from build123d import *

# Parameters (mm, degrees)
F1_DEPTH = 10.16
F3_DEPTH = 7.62


# Not quite as in the source:
# - a feature names something its author has since deleted; it is built from what else it names


with BuildPart() as f1:
    # F0 (on Top) → F1 (new body)
    with BuildSketch(Plane.XY):
        Polygon((-19.05, 19.05), (0, 0), (0, 5.2605122421), (0, 38.1), align=None)
        with BuildLine():
            Line((1.1407175417, 0), (0, 0))
            Line((0, 0), (0, -38.1))
            Line((0, -38.1), (19.05, -19.05))
            Line((19.05, -19.05), (3.7197438789, -3.7197438789))
            ThreePointArc((3.7197438789, -3.7197438789), (2.263176494, -1.9756963719), (1.1407175417, 0))
        make_face()
        Polygon((-19.05, -19.05), (0, 0), (-38.1, 0), align=None)
        Polygon((-38.1, 0), (0, 0), (-19.05, 19.05), align=None)
        Polygon((0, -38.1), (0, 0), (-19.05, -19.05), align=None)
        with BuildLine():
            Line((0, 38.1), (0, 5.2605122421))
            ThreePointArc((0, 5.2605122421), (0.2032791438, 2.9973357481), (0.8066091092, 0.8066091092))
            Line((0.8066091092, 0.8066091092), (19.05, 19.05))
            Line((19.05, 19.05), (0, 38.1))
        make_face()
        with BuildLine():
            ThreePointArc((0.8066091092, 0.8066091092), (0.9667299371, 0.4004326511), (1.1407175417, 0))
            Line((1.1407175417, 0), (38.1, 0))
            Line((38.1, 0), (19.05, 19.05))
            Line((19.05, 19.05), (0.8066091092, 0.8066091092))
        make_face()
        with BuildLine():
            Line((38.1, 0), (1.1407175417, 0))
            ThreePointArc((1.1407175417, 0), (2.263176494, -1.9756963719), (3.7197438789, -3.7197438789))
            Line((3.7197438789, -3.7197438789), (19.05, -19.05))
            Line((19.05, -19.05), (38.1, 0))
        make_face()
        Polygon((7.62, -45.72), (0, -38.1), (0, -63.5), align=None)
        Polygon((-7.62, -45.72), (0, -38.1), (-19.05, -19.05), align=None)
        Polygon((19.05, -19.05), (0, -38.1), (7.62, -45.72), align=None)
        Polygon((0, -63.5), (0, -38.1), (-7.62, -45.72), align=None)
        Polygon((-45.72, -7.62), (-38.1, 0), (-63.5, 0), align=None)
        Polygon((-45.72, 7.62), (-38.1, 0), (-19.05, 19.05), align=None)
        Polygon((-63.5, 0), (-38.1, 0), (-45.72, 7.62), align=None)
        Polygon((-19.05, -19.05), (-38.1, 0), (-45.72, -7.62), align=None)
        Polygon((-7.62, 45.72), (-19.05, 19.05), (0, 38.1), align=None)
        Polygon((-7.62, 45.72), (0, 38.1), (0, 63.5), align=None)
        Polygon((7.62, 45.72), (0, 38.1), (19.05, 19.05), align=None)
        Polygon((0, 63.5), (0, 38.1), (7.62, 45.72), align=None)
        Polygon((45.72, 7.62), (38.1, 0), (63.5, 0), align=None)
        Polygon((45.72, -7.62), (38.1, 0), (19.05, -19.05), align=None)
        Polygon((19.05, 19.05), (38.1, 0), (45.72, 7.62), align=None)
        Polygon((63.5, 0), (38.1, 0), (45.72, -7.62), align=None)
        Polygon((7.62, -45.72), (0, -63.5), (-7.62, -45.72), (-25.4, -63.5), (0, -75.1397422652), (25.4, -63.5), align=None)
        Polygon((-45.72, -7.62), (-63.5, 0), (-45.72, 7.62), (-63.5, 25.4), (-75.1397422652, 0), (-63.5, -25.4), align=None)
        Polygon((-25.4, 63.5), (-7.62, 45.72), (0, 63.5), (7.62, 45.72), (25.4, 63.5), (0, 75.1238912344), align=None)
        Polygon((45.72, 7.62), (63.5, 0), (45.72, -7.62), (63.5, -25.4), (75.1397422652, 0), (63.5, 25.4), align=None)
    extrude(amount=F1_DEPTH)

    # F2 (on face) → F3 (join)
    with BuildSketch(Plane.XY.offset(10.16)):
        Polygon((-19.05, 19.05), (-45.72, 7.62), (-45.72, -7.62), (-19.05, -19.05), (-7.62, -45.72), (7.62, -45.72), (19.05, -19.05), (45.72, -7.62), (45.72, 7.62), (19.05, 19.05), (7.62, 45.72), (-7.62, 45.72), align=None)
        Polygon((0, -30.48), (-30.48, 0), (0, 30.48), (30.48, 0), align=None, mode=Mode.SUBTRACT)
    extrude(amount=F3_DEPTH)


solid = f1.part
Input: part model. Units: mm. Frame: model coordinates. A direction names the side the tool comes from. Give positions to 0.01 mm unless a question says otherwise; leave off trailing zeros. Order: outer loops, then holes, each group sorted by start corner. A loop starts at its lowest first (then second) coordinate and runs counter-clockwise, first axis right, second up. Notation, with made-up numbers: (87, 69.25) - (116, 69.25) arc R23 cw to (116, 92.25) - close; hole circle Ø1 at (86.5, -1). An arc over 180 degrees is marked (long way). Write each question's results on one line, items separated by ' | '.
Item 1: Contact query for flat-ended pins moving along their axis: pin 1 Ø6 at (y, z) = (1.5, 3.5) entering from +X; pin 2 Ø10 at (x, y) = (-16, -2) entering from +Z; pin 3 Ø2.5 at (y, z) = (0.5, 15) entering from +X; pin 4 Ø2 at (x, z) = (54, 12) entering from +Y. Output: stop coordinate, or through.
A:
pin 1: stops at x = 75.14 | pin 2: stops at z = 10.16 | pin 3: stops at x = 45.72 | pin 4: passes through
Item 2: Section C-C (x = -55). Return loops of the section in (y, z).
A:
outline: (-16.9, 0) - (16.9, 0) - (16.9, 10.16) - (-16.9, 10.16) - close
Item 3: Section B-B (z = 8). Return loops of the section in (x, y).
A:
outline: (-75.14, 0) - (-63.5, -25.4) - (-45.72, -7.62) - (-19.05, -19.05) - (-7.62, -45.72) - (-25.4, -63.5) - (0, -75.14) - (25.4, -63.5) - (7.62, -45.72) - (19.05, -19.05) - (45.72, -7.62) - (63.5, -25.4) - (75.14, 0) - (63.5, 25.4) - (45.72, 7.62) - (19.05, 19.05) - (7.62, 45.72) - (25.4, 63.5) - (0, 75.12) - (-25.4, 63.5) - (-7.62, 45.72) - (-19.05, 19.05) - (-45.72, 7.62) - (-63.5, 25.4) - close; hole (0, 0) - (1.14, 0) arc R12.7 cw to (0, 5.26) - close
Item 4: Material intervals for line 1 along X through (y, z) = (-14, 10); line 2 along X through (y, z) = (-22.5, 8); line 3 along Y through (x, z) = (7, 11.75), sorted ascending.
A:
line 1: x = -68.72 to -52.1, -30.83 to 30.83, 52.1 to 68.72 | line 2: x = -64.83 to -60.6, -17.57 to 17.57, 60.6 to 64.83 | line 3: y = -45.72 to -23.48, 23.48 to 45.72
Item 5: Access query for faces 5 (the flat face through (-13.415, -32.198, 8.766)), 6 (the flat face through (0, 61, 10.16)), 7 (the flat face through (-54.7, -16.6, 5)), 8 (the flat face through (54.7, 16.6, 5)). Directions: +Z, -Z, +X, -X, +Y, -Y. A direction counts if a zero-diameter tool reaches every point of the face in a straight line with its end or side. Return the directions, or none.
A:
face 5: +Z, -Z | face 6: +Z, +X, -X, +Y | face 7: +Z, -Z, -Y | face 8: +Z, -Z, +Y
Item 6: Section A-A (x = -10). Return loops of the section in (y, z).
A:
outline: (-70.56, 0) - (-48.1, 0) - (-48.1, 10.16) - (-70.56, 10.16) - close; (-40.17, 0) - (40.17, 0) - (40.17, 17.78) - (20.48, 17.78) - (20.48, 10.16) - (-20.48, 10.16) - (-20.48, 17.78) - (-40.17, 17.78) - close; (48.1, 0) - (70.55, 0) - (70.55, 10.16) - (48.1, 10.16) - close
Item 7: Draft query along Y for faces 1 (the flat face through (-0.4, 0.4, 10.16)), 2 (the flat face through (16.6, -54.7, 5)), 3 (the flat face through (0, 45.72, 14)), 4 (the flat face through (45.72, 0, 14)). Return one class per face: released by +Y, released by -Y, zero draft, split by the parting line, or undercut.
A:
face 1: undercut | face 2: undercut | face 3: released by +Y | face 4: zero draft
Item 8: Section D-D (y = 54). Return loops of the section in (x, z).
A:
outline: (-15.9, 0) - (15.9, 0) - (15.9, 10.16) - (-15.9, 10.16) - close
